```python
from build123d import *

# Parameters (mm, degrees)
SKETCH_1_R      = 1.5
SKETCH_1_W      = 8.2
SKETCH_1_H      = 2.2
EXTRUDE_1_DEPTH = 2


with BuildPart() as part:
    # 草图1 → 凸台-拉伸1 (new body)
    with BuildSketch(Plane.XY):
        Polygon((-45.72603831, 61.027402263), (-45.72603831, 59.527402263), (-43.12603831, 59.527402263), (-43.12603831, 61.027402263), (-40.12603831, 61.027402263), (-40.12603831, 64.027402263), (-43.12603831, 64.027402263), (-43.12603831, 65.527402263), (-45.72603831, 65.527402263), (-45.72603831, 64.027402263), (-48.22603831, 64.027402263), (-48.22603831, 89.964902263), (-51.22603831, 89.964902263), (-51.22603831, 97.964902263), (-48.22603831, 97.964902263), (-48.22603831, 150.839902263), (-51.22603831, 150.839902263), (-51.22603831, 158.839902263), (-48.22603831, 158.839902263), (-48.22603831, 184.777402263), (-45.72603831, 184.777402263), (-45.72603831, 183.277402263), (-43.12603831, 183.277402263), (-43.12603831, 184.777402263), (-40.12603831, 184.777402263), (-40.12603831, 187.777402263), (-43.12603831, 187.777402263), (-43.12603831, 189.277402263), (-45.72603831, 189.277402263), (-45.72603831, 187.777402263), (-48.22603831, 187.777402263), (-48.22603831, 213.714902263), (-51.22603831, 213.714902263), (-51.22603831, 221.714902263), (-48.22603831, 221.714902263), (-48.22603831, 233.059504861), (52.77396169, -4.347597737), (19.52396169, -4.347597737), (-17.97603831, -4.347597737), (-48.22603831, -4.347597737), (-48.22603831, 27.089902263), (-51.22603831, 27.089902263), (-51.22603831, 35.089902263), (-48.22603831, 35.089902263), (-48.22603831, 61.027402263), align=None)
        with Locations((-33.22603831, -0.347597737)):
            Circle(SKETCH_1_R, mode=Mode.SUBTRACT)
        with Locations((32.77396169, -0.347597737)):
            Circle(SKETCH_1_R, mode=Mode.SUBTRACT)
        with Locations((-17.97603831, -0.347597737)):
            Rectangle(SKETCH_1_W, SKETCH_1_H, mode=Mode.SUBTRACT)
        with Locations((17.52396169, -0.347597737)):
            Rectangle(SKETCH_1_W, SKETCH_1_H, mode=Mode.SUBTRACT)
        with BuildLine():
            Line((-33.22603831, 158.839902263), (25.051240135, 19.790255804))
            Line((25.051240135, 19.790255804), (-29.798759865, 19.790255804))
            Line((-29.798759865, 19.790255804), (-33.22603831, 19.790255804))
            Line((-33.22603831, 19.790255804), (-33.22603831, 27.089902263))
            Line((-33.22603831, 27.089902263), (-33.22603831, 55.327402263))
            ThreePointArc((-33.22603831, 55.327402263), (-29.62603831, 62.527402263), (-33.22603831, 69.727402263))
            Line((-33.22603831, 69.727402263), (-33.22603831, 158.839902263))
        make_face(mode=Mode.SUBTRACT)
    extrude(amount=EXTRUDE_1_DEPTH)


solid = part.part
```
Can you work these out from the model? Positions are in its coordinate system, mm. Give positions to 0.01 mm unless a question says otherwise; leave off trailing zeros. Loops run counter-clockwise (first coordinate to the right, second up) from the corner with the lowest first, then second, coordinate; pieces in that order, holes last. Notation, with made-up numbers: M 80.25,86.5 L 105.25,86.5 A28 cw 105.25,122.5 Z; hole C 67,64.25 d7. An arc over 180 degrees is marked long. One line per question, with ' | ' between items. Start each with the question number.
Q1. If I drill on line 1 (Y direction, x = 19.5, z = 1.6); line 2 (Y direction, x = -1.5, z = 1.7); line 3 (Y direction, x = 42.5, z = 1.55), over which ranges is the centre line in solid material (lowest first)? Write a range as from..to.
Q2. If we section it at A-A (y = 142.5): Please give me the cut outline in (x, z).
Q3. If we section it at D-D (x = 44.5): Please give me the cut outline in (y, z), plus the area to 3 significant figures.
Q4. If we section it at B-B (x = 10.5): Please give me the cut outline in (y, z), plus the area to 3 significant figures.
Q5. For pin 1 Ø0.6 at (x, z) = (-44, 0.5) entering from +Y; pin 2 Ø1 at (x, z) = (-18.5, 1) entering from +Y; pin 3 Ø0.8 at (y, z) = (65, 1.5) entering from +X; pin 4 Ø1.8 at (x, y) = (32.77, -0.35) entering from -Z, each with a flat end and sliding along its axis, tell me the tip position at first contact or that it passes through.
Q6. If we mould it in two halves opening along Y, with no side actions, what happens to faces 1 (the flat face through (1.567, 116.018, 0.986)), 2 (the flat face through (-4.5, 90.3, 1)), 3 (the flat face through (-3, 89, 2))? For each: +Y half, -Y half, draft (parallel to the pull), parting line (faces both ways), or undercut.
Q7. If we section it at C-C (z = 1.25): State how many separate pieces and enclosed holes the cut face has, plus the area to 3 significant figures.
Computed:
1) line 1: y = -4.35..-1.45, 0.75..19.79, 33.04..73.87 | line 2: y = -4.35..19.79, 83.14..123.23 | line 3: y = -4.35..19.8
2) outline: M -48.23,0 L -33.23,0 L -33.23,2 L -48.23,2 Z; M -26.38,0 L -9.7,0 L -9.7,2 L -26.38,2 Z
3) outline: M -4.35,0 L 15.1,0 L 15.1,2 L -4.35,2 Z | area: 38.9 mm²
4) outline: M -4.35,0 L 19.79,0 L 19.79,2 L -4.35,2 Z; M 54.51,0 L 95.02,0 L 95.02,2 L 54.51,2 Z | area: 129 mm²
5) pin 1: stops at y = 223.83 | pin 2: stops at y = 164.36 | pin 3: stops at x = 23.44 | pin 4: passes through
6) face 1: +Y half | face 2: undercut | face 3: draft
7) separate pieces: 1 | enclosed holes: 5 | area: 7,960 mm²
